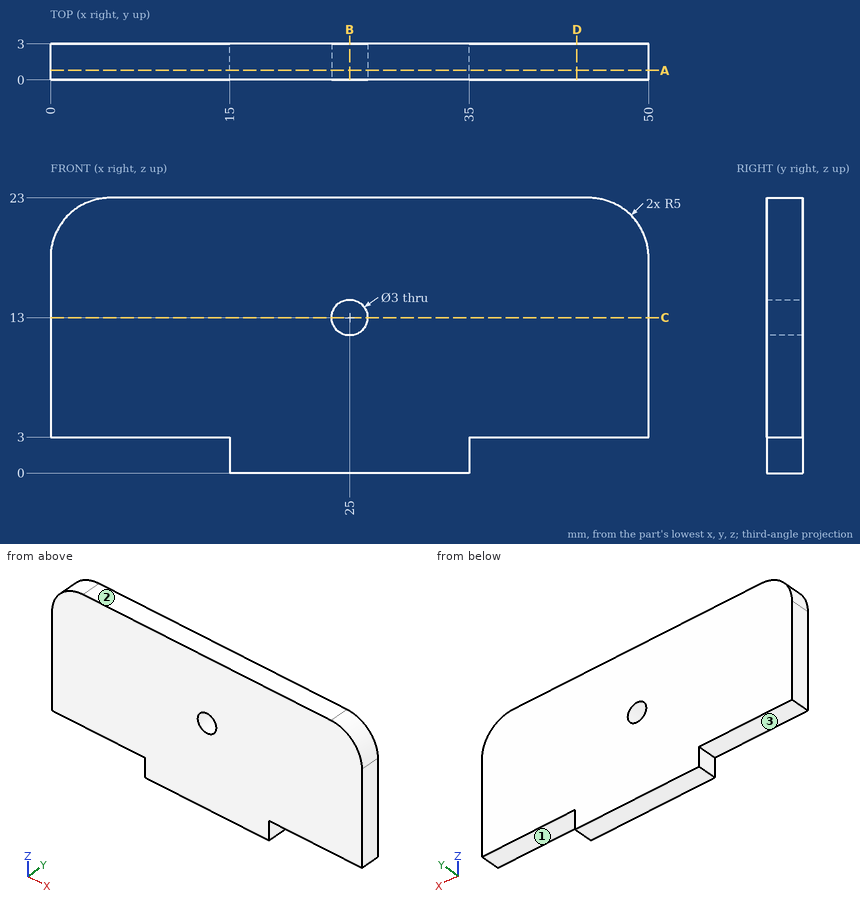
Here's the drawing with two shaded views (mm, measured from the low corner). I have some questions. A direction names the side the tool comes from. Coordinates: 2 decimals unless noted, no trailing zeros. Loops run counter-clockwise (first coordinate to the right, second up) from the corner with the lowest first, then second, coordinate; pieces in that order, holes last.
Item 1: Suppose I cut it at A-A (y = 0.8). Please give me the cut outline in (x, z).
Answers below:
outline: (0, 3) - (15, 3) - (15, 0) - (35, 0) - (35, 3) - (50, 3) - (50, 18) arc R5 ccw to (45, 23) - (5, 23) arc R5 ccw to (0, 18) - close; hole circle Ø3 at (25, 13)
Item 2: Please list where these lines run through material, in increasing order: L1, parallel to X at y = 1.7, z = 13; L2, parallel to Z at x = 8.5, y = 1.45; L3, parallel to X at y = 2.5, z = 12.5.
Answers below:
L1: x = 0 to 23.5, 26.5 to 50
L2: z = 3 to 23
L3: x = 0 to 23.59, 26.41 to 50
Item 3: I'm going to push flat-ended pins straight in: pin 1 (0.9 mm diameter, centred on y = 1, z = 1.5, fed in from +X); pin 2 (0.9 mm diameter, centred on x = 4, y = 2, fed in from -Z). Where does each tip first touch, or does it pass through?
Answers below:
pin 1: stops at x = 35
pin 2: stops at z = 3
Item 4: Suppose I cut it at B-B (x = 25). Please give me the cut outline in (y, z), then the cut area to 3 significant figures.
Answers below:
outline: (0, 0) - (3, 0) - (3, 11.5) - (0, 11.5) - close; (0, 14.5) - (3, 14.5) - (3, 23) - (0, 23) - close
area: 60.0 mm2
Item 5: Suppose I cut it at C-C (z = 13). Please give me the cut outline in (x, y), then the cut area to 3 significant figures.
Answers below:
outline: (0, 0) - (23.5, 0) - (23.5, 3) - (0, 3) - close; (26.5, 0) - (50, 0) - (50, 3) - (26.5, 3) - close
area: 141 mm2
Item 6: Suppose I cut it at D-D (x = 44). Please give me the cut outline in (y, z).
Answers below:
outline: (0, 3) - (3, 3) - (3, 23) - (0, 23) - close
Item 7: Which directions (+Z, -Z, +X, -X, +Y, -Y) give clear straight access to the entire face, cutting with the end or side of a thin tool? Please do the marked faces 1, 2 and 3.
Answers below:
face 1: -Z, +X, +Y, -Y
face 2: +Z, +X, -X, +Y, -Y
face 3: -Z, -X, +Y, -Y
